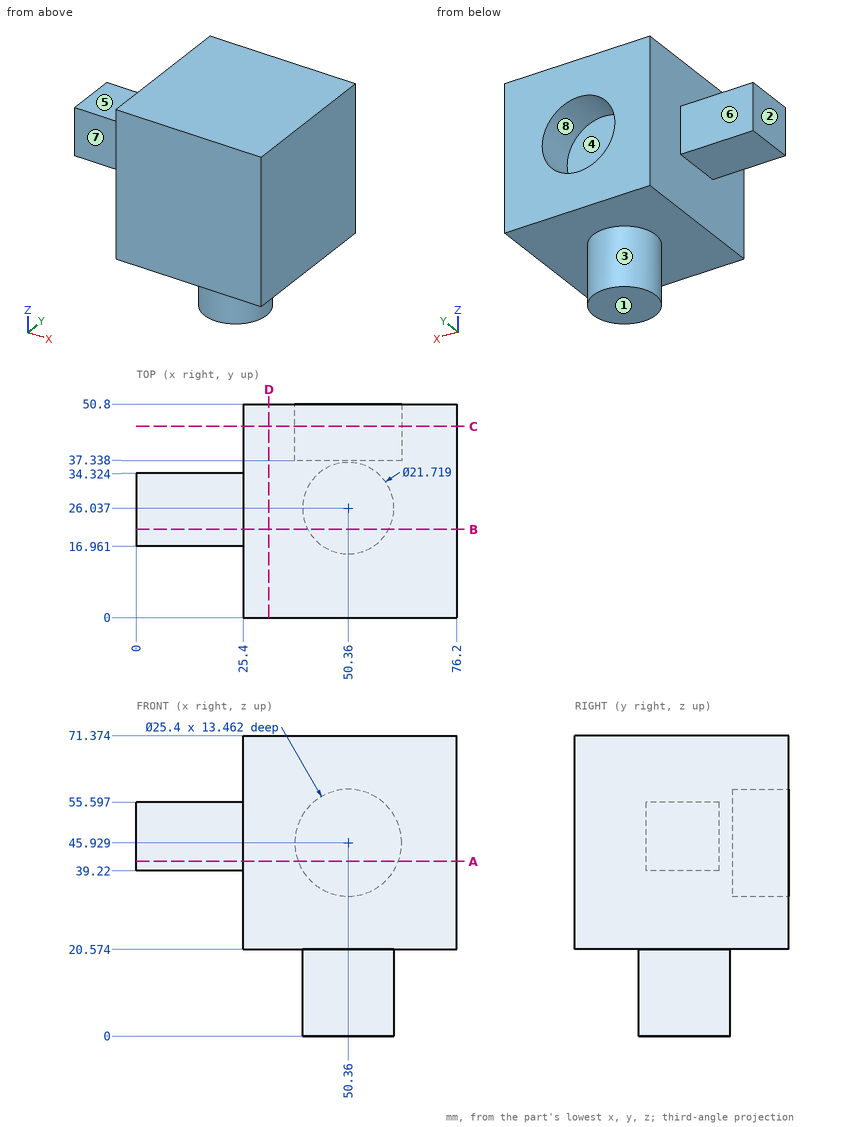
Verification items for this drawing (mm, ordinates from the low corner). A direction names the side the tool comes from. Coordinates: 2 decimals unless noted, no trailing zeros. Write each loop counter-clockwise with the first axis right and the second up, starting at its lowest first coordinate (ties: lowest second). Pieces come first, ordered by that corner, then holes. Notation, with made-up numbers: M 81.5,-3.5 L 102.5,-3.5 A11 ccw 102.5,10.5 Z; hole C 88.5,44 d8. An arc over 180 degrees is marked long. One line per item, written item: value. Start each with the question number.
(1) Scan lines: line 1 along X through (y, z) = (37, 29); line 2 along Z through (x, y) = (21, 31); line 3 along Z through (x, y) = (40, 10). Record each from-to range of solid material in increasing order. Write a range as [from, to].
(2) Sectioned sample at D-D, the plane x = 31.5. Enter the section's corners in (y, z).
(3) Depth check by flat-ended pin: pin 1 (12 mm diameter, centred on y = 35, z = 18, fed in from +X); pin 2 (8 mm diameter, centred on x = 15, z = 47.5, fed in from +Y); pin 3 (19 mm diameter, centred on x = 18.5, y = 22, fed in from -Z); pin 4 (7.5 mm diameter, centred on x = 49.5, z = 40.5, fed in from +Y). Enter the tip coordinate at first touch or a pass-through.
(4) Sectioned sample at C-C, the plane y = 45.5. Enter the section's corners in (x, z), and give its area (3 significant figures).
(5) Sectioned sample at B-B, the plane y = 21. Enter the section's corners in (x, z).
(6) Tool access check on the marked faces 5, 6, 7 and 8. Record the directions out of +Z, -Z, +X, -X, +Y, -Y that give a thin tool (end or side, any length) a straight path to the whole face; none if there is none.
(7) Sectioned sample at A-A, the plane z = 41.5. Enter the section's corners in (x, y) (1 decimal), and give its area (3 significant figures).
(8) Release check for a two-part mould opening along X. For the marked faces 1, 2, 3 and 4 record: released by +X, released by -X, zero draft, split by the parting line, or undercut.
Filled sheet:
1. line 1: [25.4, 76.2]
1. line 2: [39.22, 55.6]
1. line 3: [20.57, 71.37]
2. outline: M 0,20.57 L 50.8,20.57 L 50.8,71.37 L 0,71.37 Z
3. pin 1: x = 76.2
3. pin 2: y = 34.32
3. pin 3: z = 20.57
3. pin 4: y = 37.34
4. outline: M 25.4,20.57 L 76.2,20.57 L 76.2,71.37 L 25.4,71.37 Z; hole C 50.36,45.93 d25.4
4. area: 2,070 mm²
5. outline: M 0,39.22 L 25.4,39.22 L 25.4,20.57 L 40.74,20.57 L 40.74,0 L 59.98,0 L 59.98,20.57 L 76.2,20.57 L 76.2,71.37 L 25.4,71.37 L 25.4,55.6 L 0,55.6 Z
6. face 5: +Z, -X, +Y, -Y
6. face 6: +Z, -Z, -X, +Y
6. face 7: +Z, -Z, -X, -Y
6. face 8: +Y
7. outline: M 0,17 L 25.4,17 L 25.4,0 L 76.2,0 L 76.2,50.8 L 62.3,50.8 L 62.3,37.3 L 38.5,37.3 L 38.5,50.8 L 25.4,50.8 L 25.4,34.3 L 0,34.3 Z
7. area: 2,700 mm²
8. face 1: zero draft
8. face 2: released by -X
8. face 3: split by the parting line
8. face 4: undercut
